from build123d import *

# Parameters (mm, degrees)
SKETCH1_W                = 120
SKETCH1_H                = 30
BOSS_EXTRUDE1_DEPTH      = 100
CUT_EXTRUDE1_DEPTH       = 121.415945788
CUT_EXTRUDE1_DEPTH_BACK  = 121.415945788
SKETCH2_R                = 2.15
SKETCH2_W                = 20.1
SKETCH2_H                = 40.4
SKETCH3_OUTSIDE_W        = 153.812
SKETCH3_OUTSIDE_H        = 133.812
CUT_EXTRUDE2_DEPTH       = 121.415945788
CUT_EXTRUDE3_START       = -30
CUT_EXTRUDE3_DEPTH       = 30
SKETCH5_W                = 67.698745078
SKETCH5_H                = 100.8
CUT_EXTRUDE4_DEPTH       = 26
RIB1_REACH               = 122.416
SKETCH6_WALL_W           = 284.590065176
SKETCH6_WALL_H           = 4
RIB6_REACH               = 122.416
SKETCH7_WALL_W           = 284.590065176
SKETCH7_WALL_H           = 4
BOSS_EXTRUDE2_DEPTH      = 5
BOSS_EXTRUDE2_DEPTH_BACK = 4
SKETCH8_R                = 2.15
CUT_EXTRUDE5_DEPTH       = 84.326168543
CUT_EXTRUDE5_DEPTH_BACK  = 84.326168543
SKETCH9_R                = 2.75
SKETCH10_R               = 5
CUT_EXTRUDE6_DEPTH       = 3
CHAMFER1_SIZE            = 8
CUT_EXTRUDE7_START       = -12.194246874
CUT_EXTRUDE7_DEPTH       = 12.194246874


# Read off the part's stored shape, not the designer's step: Cut-Extrude3, Cut-Extrude7
with BuildPart() as part:
    # Sketch1 → Boss-Extrude1 (new body)
    with BuildSketch(Plane(origin=(0, 0, 0), x_dir=(1, 0, 0), z_dir=(0, 1, 0))):
        with Locations((0, -15)):
            Rectangle(SKETCH1_W, SKETCH1_H)
    extrude(amount=BOSS_EXTRUDE1_DEPTH)

    # Sketch2 → Cut-Extrude1 (cut, two sides: drawn at the far end of the back side and taken through both)
    with BuildSketch(Plane.XY.offset(30).offset(-CUT_EXTRUDE1_DEPTH_BACK)):
        with Locations((-4.95, 82.583541889)):
            Circle(SKETCH2_R)
        with Locations((4.95, 82.583541889)):
            Circle(SKETCH2_R)
        with Locations((-4.95, 34.383541889)):
            Circle(SKETCH2_R)
        with Locations((4.95, 34.383541889)):
            Circle(SKETCH2_R)
        with Locations((0, 58.483541889)):
            Rectangle(SKETCH2_W, SKETCH2_H)
    extrude(amount=CUT_EXTRUDE1_DEPTH + CUT_EXTRUDE1_DEPTH_BACK, mode=Mode.SUBTRACT)

    # Sketch3 outside → Cut-Extrude2 (cut, through all)
    with BuildSketch(Plane.XY.offset(30)):
        with Locations((0, 50)):
            Rectangle(SKETCH3_OUTSIDE_W, SKETCH3_OUTSIDE_H)
        with BuildLine():
            Line((-45, 23.283541889), (45, 23.283541889))
            Line((45, 23.283541889), (19.804596008, 86.568297014))
            ThreePointArc((19.804596008, 86.568297014), (0, 100), (-19.804596008, 86.568297014))
            Line((-19.804596008, 86.568297014), (-45, 23.283541889))
        make_face(mode=Mode.SUBTRACT)
    extrude(amount=-CUT_EXTRUDE2_DEPTH, mode=Mode.SUBTRACT)

    # Cut-Extrude3 outline → Cut-Extrude3 (cut)
    with BuildSketch(Plane.XY.offset(30).offset(CUT_EXTRUDE3_START)):
        Polygon((30, 60.95991045), (30, 23.283541889), (45, 23.283541889), align=None)
        Polygon((-30, 23.283541889), (-30, 60.95991045), (-45, 23.283541889), align=None)
    extrude(amount=CUT_EXTRUDE3_DEPTH, mode=Mode.SUBTRACT)

    # Sketch5 → Cut-Extrude4 (cut)
    with BuildSketch(Plane.XY.offset(30)):
        with Locations((0, 78.683541889)):
            Rectangle(SKETCH5_W, SKETCH5_H)
    extrude(amount=-CUT_EXTRUDE4_DEPTH, mode=Mode.SUBTRACT)

    # Sketch6 wall → Rib1 (add, up to next)
    with BuildSketch(Plane(origin=(-30, 44.62172617, 17), x_dir=(0, -0.782514313837, 0.622632595228), z_dir=(0, 0.622632595228, 0.782514313837)), mode=Mode.PRIVATE) as rib1_sk1:
        with Locations((0, 2)):
            Rectangle(SKETCH6_WALL_W, SKETCH6_WALL_H)
    rib1_tool1 = extrude(rib1_sk1.sketch, amount=-RIB1_REACH, mode=Mode.PRIVATE) - part.part
    add(rib1_tool1.solids().sort_by_distance((-30, 44.62172617, 17))[0])

    # Sketch7 wall → Rib6 (add, up to next)
    with BuildSketch(Plane(origin=(30, 44.62172617, 17), x_dir=(0, -0.782514313837, 0.622632595228), z_dir=(0, -0.622632595228, -0.782514313837)), mode=Mode.PRIVATE) as rib6_sk1:
        with Locations((0, 2)):
            Rectangle(SKETCH7_WALL_W, SKETCH7_WALL_H)
    rib6_tool1 = extrude(rib6_sk1.sketch, amount=RIB6_REACH, mode=Mode.PRIVATE) - part.part
    add(rib6_tool1.solids().sort_by_distance((30, 44.62172617, 17))[0])

    # Sketch8 → Boss-Extrude2 (add, two sides: drawn at the far end of the back side and taken through both)
    with BuildSketch(Plane.XY.offset(4).offset(-BOSS_EXTRUDE2_DEPTH_BACK)):
        with Locations((-4.95, 82.583541889)):
            Circle(SKETCH8_R)
        with Locations((4.95, 82.583541889)):
            Circle(SKETCH8_R)
        with Locations((-4.95, 34.383541889)):
            Circle(SKETCH8_R)
        with Locations((4.95, 34.383541889)):
            Circle(SKETCH8_R)
    extrude(amount=BOSS_EXTRUDE2_DEPTH + BOSS_EXTRUDE2_DEPTH_BACK)

    # Sketch9 → Cut-Extrude5 (cut, two sides: drawn at the far end of the back side and taken through both)
    with BuildSketch(Plane(origin=(0, 28.283541889, 0), x_dir=(1, 0, 0), z_dir=(0, 1, 0)).offset(-CUT_EXTRUDE5_DEPTH_BACK)):
        with Locations(Location((-15, -15, 0), (0, 0, 270))):
            Circle(SKETCH9_R)
        with Locations(Location((15, -15, 0), (0, 0, 270))):
            Circle(SKETCH9_R)
    extrude(amount=CUT_EXTRUDE5_DEPTH + CUT_EXTRUDE5_DEPTH_BACK, mode=Mode.SUBTRACT)

    # Sketch10 → Cut-Extrude6 (cut)
    with BuildSketch(Plane(origin=(0, 28.283541889, 0), x_dir=(1, 0, 0), z_dir=(0, 1, 0))):
        with Locations(Location((-15, -15, 0), (0, 0, 270))):
            Circle(SKETCH10_R)
        with Locations(Location((15, -15, 0), (0, 0, 270))):
            Circle(SKETCH10_R)
    extrude(amount=-CUT_EXTRUDE6_DEPTH, mode=Mode.SUBTRACT)

    # Chamfer1
    # the kernel refuses this chamfer: 8 mm, written as the material it takes off along each edge
    with BuildSketch(Plane(origin=(-30, 2.710077985, 30), x_dir=(-0.02749587661058658, 0, -0.9996219169112968), z_dir=(0, 1, 0))) as chamfer1_piece_1:
        Polygon((CHAMFER1_SIZE * 0.999621916911, -CHAMFER1_SIZE * 0.0274958766106), (-CHAMFER1_SIZE * 0.0274958766106, -CHAMFER1_SIZE * 0.999621916911), (0, 0), align=None)
    extrude(amount=46.146927807, mode=Mode.SUBTRACT)
    with BuildSketch(Plane(origin=(30, 48.857005793, 30), x_dir=(-0.9996219169112968, 0, 0.027495876610586487), z_dir=(0, -1, 0))) as chamfer1_piece_2:
        Polygon((CHAMFER1_SIZE * 0.999621916911, CHAMFER1_SIZE * 0.0274958766106), (-CHAMFER1_SIZE * 0.0274958766106, CHAMFER1_SIZE * 0.999621916911), (0, 0), align=None)
    extrude(amount=46.146927807, mode=Mode.SUBTRACT)

    # Cut-Extrude7 outline → Cut-Extrude7 (cut)
    with BuildSketch(Plane.XZ.offset(-23.283541889).offset(CUT_EXTRUDE7_START)):
        with BuildLine():
            ThreePointArc((-27.724333118, 24.275666882), (-14.154563191, 28.553981218), (0, 30))
            Line((0, 30), (-22, 30))
            Line((-22, 30), (-27.724333118, 24.275666882))
        make_face()
        with BuildLine():
            ThreePointArc((0, 30), (14.154563191, 28.553981218), (27.724333118, 24.275666882))
            Line((27.724333118, 24.275666882), (22, 30))
            Line((22, 30), (0, 30))
        make_face()
    extrude(amount=CUT_EXTRUDE7_DEPTH, mode=Mode.SUBTRACT)


solid = part.part
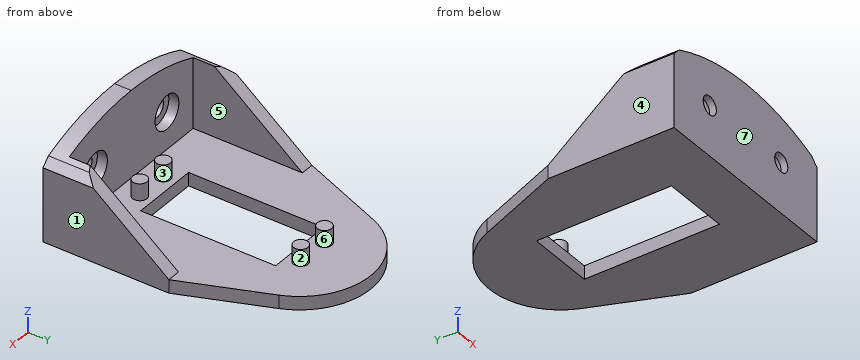
Verification items for the finished model (mm, model axes). Face numbers are marked on the shaded views. A direction names the side the tool comes from. Round coordinates to 2 decimals unless told otherwise and drop trailing zeros. Order: outer loops, then holes, each group sorted by start corner. A loop starts at its lowest first (then second) coordinate and runs counter-clockwise, first axis right, second up.
1. Section check B-B on x = 4.95. Record the cut outline in (y, z).
Final values:
outline: (23.28, 0) - (38.28, 0) - (38.28, 4) - (36.53, 4) - (36.53, 9) - (32.23, 9) - (32.23, 4) - (28.28, 4) - (28.28, 29.82) - (23.28, 29.82) - close; (78.68, 0) - (99.42, 0) - (99.42, 4) - (84.73, 4) - (84.73, 9) - (80.43, 9) - (80.43, 4) - (78.68, 4) - close
2. Access from +Z, -Z, +X, -X, +Y, -Y to the whole of each face (thin tool, end or side, straight path). Record for the marked faces 5, 6 and 7.
Final values:
face 5: +Z, +Y
face 6: +Z
face 7: +Z, -Z, +X, -X, -Y
3. Go/stop test with flat-tipped pins: P1, Ø17, axis at y = 45, z = 17.5, coming from the -X side; P2, Ø3, axis at x = 15.5, z = 16, coming from the +Y side; P3, Ø11, axis at x = 16, z = 16, coming from the +Y side; P4, Ø4.5, axis at x = -5.5, y = 34, coming from the +Z side. Record where each tip stops, or that it passes through.
Final values:
P1: stops at x = -30
P2: passes through
P3: stops at y = 28.28
P4: stops at z = 9
4. Release check for a two-part mould opening along X. For the marked faces 1, 2, 3 and 4 record: +X half, -X half, draft (parallel to the pull), parting line (faces both ways), or undercut.
Final values:
face 1: +X half
face 2: undercut
face 3: undercut
face 4: -X half
5. Section check D-D on z = 7. Record the cut outline in (x, y), then the cut area to 3 significant figures.
Final values:
outline: (-30, 23.28) - (30, 23.28) - (30, 57.19) - (26, 57.19) - (26, 28.28) - (-26, 28.28) - (-26, 57.19) - (-30, 57.19) - close; circle Ø4.3 at (-4.95, 34.38); circle Ø4.3 at (-4.95, 82.58); circle Ø4.3 at (4.95, 34.38); circle Ø4.3 at (4.95, 82.58)
area: 589 mm2
6. Section check C-C on y = 73. Record the cut outline in (x, z).
Final values:
outline: (-25.21, 0) - (-10.05, 0) - (-10.05, 4) - (-25.21, 4) - close; (10.05, 0) - (25.21, 0) - (25.21, 4) - (10.05, 4) - close
7. Section check A-A on z = 15. Record the cut outline in (x, y), then the cut area to 3 significant figures.
Final values:
outline: (-30, 23.28) - (-17.75, 23.28) - (-17.75, 25.28) - (-20, 25.28) - (-20, 28.28) - (-26, 28.28) - (-26, 47.14) - (-30, 47.14) - close; (-12.25, 23.28) - (12.25, 23.28) - (12.25, 25.28) - (10, 25.28) - (10, 28.28) - (-10, 28.28) - (-10, 25.28) - (-12.25, 25.28) - close; (17.75, 23.28) - (30, 23.28) - (30, 47.14) - (26, 47.14) - (26, 28.28) - (20, 28.28) - (20, 25.28) - (17.75, 25.28) - close
area: 369 mm2
8. Thickness scan on L1, parallel to X at y = 26.7, z = 15; L2, parallel to X at y = 24.7, z = 15; L3, parallel to X at y = 37, z = 14.5. Record the ranges inside material, lowest first.
Final values:
L1: x = -30 to -20, -10 to 10, 20 to 30
L2: x = -30 to -17.75, -12.25 to 12.25, 17.75 to 30
L3: x = -30 to -26, 26 to 30
